from build123d import *

# Parameters (mm, degrees)
SKETCH1_R           = 0.8
BOSS_EXTRUDE1_DEPTH = 3
FILLET1_R           = 1


with BuildPart() as part:
    # Sketch1 → Boss-Extrude1 (new body)
    with BuildSketch(Plane.XY):
        Polygon((5, -2), (9, -2), (9, 2), (5, 2), (5, 1.5), (-5, 1.5), (-5, 2), (-9, 2), (-9, -2), (-5, -2), (-5, -1.5), (5, -1.5), align=None)
        with Locations((-7, 0)):
            Circle(SKETCH1_R, mode=Mode.SUBTRACT)
        with Locations((7, 0)):
            Circle(SKETCH1_R, mode=Mode.SUBTRACT)
    extrude(amount=BOSS_EXTRUDE1_DEPTH)

    # Fillet1
    # the kernel refuses this fillet: 1 mm, written as the material it takes off along each edge
    with BuildSketch(Plane(origin=(5, -2, -2.165063509), x_dir=(1, 0, 0), z_dir=(0, 0, 1))) as fillet1_piece_1:
        with BuildLine():
            CenterArc((0.866025404, 1), FILLET1_R, 210, 60)
            Line((0, 0.5), (-0.017320508, 0.49))
            ThreePointArc((-0.017320508, 0.49), (-0.02, 0.25), (-0.02, 0))
            Line((-0.02, 0), (0, -0.02))
            Line((0, -0.02), (0.866025404, -0.02))
            Line((0.866025404, -0.02), (0.866025404, 0))
        make_face()
    extrude(amount=7.330127019, mode=Mode.SUBTRACT)
    with BuildSketch(Plane(origin=(9, -2, -2.5), x_dir=(-1, 0, 0), z_dir=(0, 0, 1)), Plane(origin=(9, 2, -2.5), x_dir=(0, -1, 0), z_dir=(0, 0, 1)), Plane(origin=(-9, -2, -2.5), x_dir=(0, 1, 0), z_dir=(0, 0, 1)), Plane(origin=(-9, 2, -2.5), x_dir=(1, 0, 0), z_dir=(0, 0, 1))) as fillet1_piece_2:
        with BuildLine():
            CenterArc((FILLET1_R, -FILLET1_R), FILLET1_R, 90, 90)
            Line((0, -FILLET1_R), (-FILLET1_R * 0.02, -FILLET1_R))
            Line((-FILLET1_R * 0.02, -FILLET1_R), (-FILLET1_R * 0.02, FILLET1_R * 0.02))
            Line((-FILLET1_R * 0.02, FILLET1_R * 0.02), (FILLET1_R, FILLET1_R * 0.02))
            Line((FILLET1_R, FILLET1_R * 0.02), (FILLET1_R, 0))
        make_face()
    extrude(amount=8, mode=Mode.SUBTRACT)
    with BuildSketch(Plane(origin=(5, 2, -2.165063509), x_dir=(1, 0, 0), z_dir=(0, 0, 1)), Plane(origin=(-5, -2, -2.165063509), x_dir=(-1, 0, 0), z_dir=(0, 0, 1))) as fillet1_piece_3:
        with BuildLine():
            CenterArc((0.866025404, -1), FILLET1_R, 90, 60)
            Line((0, -0.5), (-0.017320508, -0.49))
            ThreePointArc((-0.017320508, -0.49), (-0.02, -0.25), (-0.02, 0))
            Line((-0.02, 0), (0, 0.02))
            Line((0, 0.02), (0.866025404, 0.02))
            Line((0.866025404, 0.02), (0.866025404, 0))
        make_face()
    extrude(amount=7.330127019, mode=Mode.SUBTRACT)
    with BuildSketch(Plane(origin=(-5, 2, -2.165063509), x_dir=(0, -1, 0), z_dir=(0, 0, 1))) as fillet1_piece_4:
        with BuildLine():
            CenterArc((1, -0.866025404), FILLET1_R, 120, 60)
            Line((0, -0.866025404), (-0.02, -0.866025404))
            Line((-0.02, -0.866025404), (-0.02, 0))
            Line((-0.02, 0), (0, 0.02))
            ThreePointArc((0, 0.02), (0.25, 0.02), (0.49, 0.017320508))
            Line((0.49, 0.017320508), (0.5, 0))
        make_face()
    extrude(amount=7.330127019, mode=Mode.SUBTRACT)


solid = part.part
Can you work these out from the model? Positions are in its coordinate system, mm. A direction names the side the tool comes from. Round coordinates to 2 decimals unless told otherwise and drop trailing zeros. Order: outer loops, then holes, each group sorted by start corner. A loop starts at its lowest first (then second) coordinate and runs counter-clockwise, first axis right, second up. Notation, with made-up numbers: (-40, 69.5) -> (-10, 69.5) arc R21 cw to (-10, 102.5) -> close; hole circle Ø6 at (87.5, 8). An arc over 180 degrees is marked (long way). Write each question's results on one line, items separated by ' | '. Start each with the question number.
Item 1: Will these pins go through, and if not, where does the flat tip stop? pin 1 (1 mm diameter, centred on x = 7, y = 0, fed in from +Z); pin 2 (1.5 mm diameter, centred on x = -2.5, y = 1.5, fed in from -Z); pin 3 (1.5 mm diameter, centred on x = 0, z = 1.5, fed in from -Y).
Item 2: If we section it at A-A, the plane x = 7: Write out the boundary of the cut face in (y, z).
Item 3: Which directions (+Z, -Z, +X, -X, +Y, -Y) give clear straight access to the entire face, cutting with the end or side of a thin tool? Please do faces 1 (the cylindrical face through (5.36, -1.862, 1.479)), 2 (the cylindrical face through (-7.8, 0, 1.5)), 3 (the cylindrical face through (5.37, 1.87, 1.48)).
Item 4: If we section it at D-D, the plane x = -0.75: Write out the boundary of the cut face in (y, z).
Item 5: If we section it at B-B, the plane y = 0: Write out the boundary of the cut face in (x, z), then the cut area to 3 significant figures.
Item 6: Thinking about a two-plate mould opening in X: for faces 4 (the flat face through (0, -1.5, 1)), 5 (the cylindrical face through (8.715, 1.699, 1.479)), 6 (the cylindrical face through (-8.699, 1.715, 1.479)), which applies, +X half, -X half, draft (parallel to the pull), parting line (faces both ways), or undercut?
Item 7: Please list where these lines run through material, in increasing order: L1, parallel to Y at x = 7, z = 1; L2, parallel to X at y = 0.2, z = 0.55; L3, parallel to X at y = -0.4, z = 0.75.
Item 8: If we section it at C-C, the plane z = 2.8: Write out the boundary of the cut face in (x, y), then the cut area to 3 significant figures.
Results:
1) pin 1: passes through | pin 2: stops at z = 0 | pin 3: stops at y = -1.5
2) outline: (-2, 0) -> (-0.8, 0) -> (-0.8, 3) -> (-2, 3) -> close; (0.8, 0) -> (2, 0) -> (2, 3) -> (0.8, 3) -> close
3) face 1: +Z, -Z, -Y | face 2: +Z, -Z | face 3: +Z, -Z, +Y
4) outline: (-1.5, 0) -> (1.5, 0) -> (1.5, 3) -> (-1.5, 3) -> close
5) outline: (-9, 0) -> (-7.8, 0) -> (-7.8, 3) -> (-9, 3) -> close; (-6.2, 0) -> (6.2, 0) -> (6.2, 3) -> (-6.2, 3) -> close; (7.8, 0) -> (9, 0) -> (9, 3) -> (7.8, 3) -> close | area: 44.4 mm2
6) face 4: undercut | face 5: +X half | face 6: -X half
7) L1: y = -2 to -0.8, 0.8 to 2 | L2: x = -9 to -7.77, -6.23 to 6.23, 7.77 to 9 | L3: x = -9 to -7.69, -6.31 to 6.31, 7.69 to 9
8) outline: (-9, -1) arc R1 ccw to (-8, -2) -> (-5.87, -2) arc R1 ccw to (-5, -1.5) -> (5, -1.5) arc R1 ccw to (5.87, -2) -> (8, -2) arc R1 ccw to (9, -1) -> (9, 1) arc R1 ccw to (8, 2) -> (5.87, 2) arc R1 ccw to (5, 1.5) -> (-5, 1.5) arc R1 ccw to (-5.87, 2) -> (-8, 2) arc R1 ccw to (-9, 1) -> close; hole circle Ø1.6 at (-7, 0); hole circle Ø1.6 at (7, 0) | area: 56.6 mm2
